Geometry check sheet. Reference: the model listing, model coordinates, mm. A direction names the side the tool comes from. Round coordinates to 2 decimals unless told otherwise and drop trailing zeros. Write each loop counter-clockwise with the first axis right and the second up, starting at its lowest first coordinate (ties: lowest second). Pieces come first, ordered by that corner, then holes. Notation, with made-up numbers: (82, 74) -> (98, 74) arc R28 cw to (98, 95) -> close; hole circle Ø9 at (21, -28.5). An arc over 180 degrees is marked (long way). Use a Markdown table: item, result.
```python
from build123d import *

# Parameters (mm, degrees)
F0_R     = 2.286
F1_DEPTH = 5.08


with BuildPart() as f1:
    # F0 (on Top) → F1 (new body)
    with BuildSketch(Plane.XY):
        with BuildLine():
            ThreePointArc((-16.394592, 8.088413), (-4.15277, -17.803359), (18.281277, 0))
            ThreePointArc((18.281277, 0), (17.803359, 4.15277), (16.394592, 8.088413))
            ThreePointArc((16.394592, 8.088413), (13.614491, 12.200439), (9.830724, 15.413044))
            ThreePointArc((9.830724, 15.413044), (0, 18.281277), (-9.830724, 15.413044))
            ThreePointArc((-9.830724, 15.413044), (-13.614491, 12.200439), (-16.394592, 8.088413))
        make_face()
        with BuildLine():
            ThreePointArc((11.172347, -3.07006), (0, -8.290545), (-11.172347, -3.07006))
            ThreePointArc((-11.172347, -3.07006), (-6.145377, -5.255343), (-0.75922, -6.272794))
            Line((-0.75922, -6.272794), (-0.75922, 0))
            Line((-0.75922, 0), (-2.770182, 2.295201))
            Line((-2.770182, 2.295201), (2.770182, 2.295201))
            Line((2.770182, 2.295201), (0.75922, 0))
            Line((0.75922, 0), (0.75922, -6.272794))
            ThreePointArc((0.75922, -6.272794), (6.145377, -5.255343), (11.172347, -3.07006))
        make_face(mode=Mode.SUBTRACT)
        with Locations((-5.628771, 8.630777)):
            Circle(F0_R, mode=Mode.SUBTRACT)
        with Locations((5.628771, 8.630777)):
            Circle(F0_R, mode=Mode.SUBTRACT)
        with BuildLine():
            ThreePointArc((9.830724, 15.413044), (13.614491, 12.200439), (16.394592, 8.088413))
            Line((16.394592, 8.088413), (19.790254, 26.43105))
            Line((19.790254, 26.43105), (9.830724, 15.413044))
        make_face()
        with BuildLine():
            Line((-19.790254, 26.43105), (-16.394592, 8.088413))
            ThreePointArc((-16.394592, 8.088413), (-13.614491, 12.200439), (-9.830724, 15.413044))
            Line((-9.830724, 15.413044), (-19.790254, 26.43105))
        make_face()
    extrude(amount=F1_DEPTH)


solid = f1.part
```
(1) Section check C-C on z = 4.6. Record the cut outline in (x, y).
A:
| item | result |
|---|---|
| outline | (-19.79, 26.43) -> (-16.39, 8.09) arc R18.28 ccw (long way) to (18.28, 0) arc R18.28 ccw to (16.39, 8.09) -> (19.79, 26.43) -> (9.83, 15.41) arc R18.28 ccw to (-9.83, 15.41) -> close; hole (-11.17, -3.07) arc R14.57 ccw to (11.17, -3.07) arc R24.59 cw to (0.76, -6.27) -> (0.76, 0) -> (2.77, 2.3) -> (-2.77, 2.3) -> (-0.76, 0) -> (-0.76, -6.27) arc R24.59 cw to start; hole circle Ø4.57 at (-5.63, 8.63); hole circle Ø4.57 at (5.63, 8.63) |
(2) Thickness scan on line 1 (Y direction, x = -2.5, z = 0.4); line 2 (Y direction, x = -1.5, z = 0.9); line 3 (X direction, y = 15.5, z = 3.1). Record the ranges inside material, lowest first.
A:
| item | result |
|---|---|
| line 1 | y = -18.11 to -8.07, -6.08 to 1.99, 2.3 to 18.11 |
| line 2 | y = -18.22 to -8.21, -6.21 to 0.85, 2.3 to 18.22 |
| line 3 | x = -17.77 to -9.91, -9.69 to 9.69, 9.91 to 17.77 |
(3) Section check D-D on y = -4.5. Record the cut outline in (x, z), plus the area to 3 significant figures.
A:
| item | result |
|---|---|
| outline | (-17.72, 0) -> (-9.8, 0) -> (-9.8, 5.08) -> (-17.72, 5.08) -> close; (-8.25, 0) -> (-0.76, 0) -> (-0.76, 5.08) -> (-8.25, 5.08) -> close; (0.76, 0) -> (8.25, 0) -> (8.25, 5.08) -> (0.76, 5.08) -> close; (9.8, 0) -> (17.72, 0) -> (17.72, 5.08) -> (9.8, 5.08) -> close |
| area | 157 mm2 |
(4) Section check A-A on x = 0. Record the cut outline in (y, z), plus the area to 3 significant figures.
A:
| item | result |
|---|---|
| outline | (-18.28, 0) -> (-8.29, 0) -> (-8.29, 5.08) -> (-18.28, 5.08) -> close; (2.3, 0) -> (18.28, 0) -> (18.28, 5.08) -> (2.3, 5.08) -> close |
| area | 132 mm2 |
(5) Access from +Z, -Z, +X, -X, +Y, -Y to the whole of each face (thin tool, end or side, straight path). Record for faces 4 (the face through (-18.116, 17.388, 2.504)), 5 (the face through (18.07, 17.13, 2.5)), 6 (the face through (-0.759, -3, 3)), 7 (the face through (-14.7, 20.8, 2.5)).
A:
| item | result |
|---|---|
| face 4 | +Z, -Z, -X |
| face 5 | +Z, -Z, +X |
| face 6 | +Z, -Z |
| face 7 | +Z, -Z, +Y |
(6) Release check for a two-part mould opening along X. For faces 1 (the face through (0, 4, 5.08)), 2 (the face through (-4.6, -17.693, 2.504)), 3 (the face through (-6.12, 6.4, 2.5)) record: +X half, -X half, draft (parallel to the pull), parting line (faces both ways), or undercut.
A:
| item | result |
|---|---|
| face 1 | draft |
| face 2 | parting line |
| face 3 | undercut |
(7) Gauge pin test, flat ends, axial feed: pin 1 Ø2 at (y, z) = (11.5, 1) entering from +X; pin 2 Ø3 at (x, z) = (-3, 2.5) entering from +Y; pin 3 Ø4 at (x, y) = (-5.63, 8.63) entering from +Z; pin 4 Ø1.5 at (y, z) = (-4.5, 1.5) entering from -X. Record the tip position at first contact, or that the pin passes through.
A:
| item | result |
|---|---|
| pin 1 | stops at x = 17.21 |
| pin 2 | stops at y = 18.22 |
| pin 3 | passes through |
| pin 4 | stops at x = -17.89 |
(8) Section check B-B on y = 16. Record the cut outline in (x, z), plus the area to 3 significant figures.
A:
| item | result |
|---|---|
| outline | (-17.86, 0) -> (-10.36, 0) -> (-10.36, 5.08) -> (-17.86, 5.08) -> close; (-8.84, 0) -> (8.84, 0) -> (8.84, 5.08) -> (-8.84, 5.08) -> close; (10.36, 0) -> (17.86, 0) -> (17.86, 5.08) -> (10.36, 5.08) -> close |
| area | 166 mm2 |
